The model under review builds one solid part; all positions refer to its coordinate system, in mm. A direction names the side the tool comes from. Give positions to 0.01 mm unless a question says otherwise; leave off trailing zeros. Loops run counter-clockwise (first coordinate to the right, second up) from the corner with the lowest first, then second, coordinate; pieces in that order, holes last. Notation, with made-up numbers: (-22, -33) - (4, -33) arc R17 ccw to (4, -25) - close; hole circle Ø1 at (22.5, -35). An arc over 180 degrees is marked (long way). Answer as a JSON object with one key per item and string values.
from build123d import *

# Parameters (mm, degrees)
SKETCH1_R           = 2.1
SKETCH1_R_2         = 2.6
BOSS_EXTRUDE1_DEPTH = 4


with BuildPart() as part:
    # Sketch1 → Boss-Extrude1 (new body)
    with BuildSketch(Plane(origin=(0, 0, 0), x_dir=(-1, 0, 0), z_dir=(0, 0, -1))):
        with BuildLine():
            Line((87.42535625, -29.106339063), (52.57464375, -20.393660937))
            ThreePointArc((52.57464375, -20.393660937), (47.11794562, -16.84635803), (45, -10.692235936))
            Line((45, -10.692235936), (45, -8))
            ThreePointArc((45, -8), (44.853553391, -7.646446609), (44.5, -7.5))
            Line((44.5, -7.5), (38, -7.5))
            ThreePointArc((38, -7.5), (37.646446609, -7.353553391), (37.5, -7))
            Line((37.5, -7), (37.5, 3))
            ThreePointArc((37.5, 3), (37.646446609, 3.353553391), (38, 3.5))
            Line((38, 3.5), (39.5, 3.5))
            ThreePointArc((39.5, 3.5), (39.853553391, 3.353553391), (40, 3))
            Line((40, 3), (40, -4.5))
            ThreePointArc((40, -4.5), (40.146446609, -4.853553391), (40.5, -5))
            Line((40.5, -5), (44.5, -5))
            ThreePointArc((44.5, -5), (44.853553391, -4.853553391), (45, -4.5))
            Line((45, -4.5), (45, 38.692235936))
            ThreePointArc((45, 38.692235936), (47.11794562, 44.84635803), (52.57464375, 48.393660937))
            Line((52.57464375, 48.393660937), (87.42535625, 57.106339063))
            ThreePointArc((87.42535625, 57.106339063), (92.88205438, 60.65364197), (95, 66.807764064))
            Line((95, 66.807764064), (95, 85))
            ThreePointArc((95, 85), (92.071067812, 92.071067812), (85, 95))
            Line((85, 95), (80.600023778, 95))
            ThreePointArc((80.600023778, 95), (75.38177505, 94.307249421), (70.525020806, 92.276988022))
            ThreePointArc((70.525020806, 92.276988022), (0, 73.215904175), (-70.525020806, 92.276988022))
            ThreePointArc((-70.525020806, 92.276988022), (-75.38177505, 94.307249421), (-80.600023778, 95))
            Line((-80.600023778, 95), (-85, 95))
            ThreePointArc((-85, 95), (-92.071067812, 92.071067812), (-95, 85))
            Line((-95, 85), (-95, 57.30993956))
            ThreePointArc((-95, 57.30993956), (-93.292887614, 51.721736358), (-88.754396995, 48.041471336))
            Line((-88.754396995, 48.041471336), (-51.245603005, 32.847708996))
            ThreePointArc((-51.245603005, 32.847708996), (-46.707112386, 29.167443975), (-45, 23.579240773))
            Line((-45, 23.579240773), (-45, -4.5))
            ThreePointArc((-45, -4.5), (-44.853553391, -4.853553391), (-44.5, -5))
            Line((-44.5, -5), (-40.5, -5))
            ThreePointArc((-40.5, -5), (-40.146446609, -4.853553391), (-40, -4.5))
            Line((-40, -4.5), (-40, 3))
            ThreePointArc((-40, 3), (-39.853553391, 3.353553391), (-39.5, 3.5))
            Line((-39.5, 3.5), (-38, 3.5))
            ThreePointArc((-38, 3.5), (-37.646446609, 3.353553391), (-37.5, 3))
            Line((-37.5, 3), (-37.5, -7))
            ThreePointArc((-37.5, -7), (-37.646446609, -7.353553391), (-38, -7.5))
            Line((-38, -7.5), (-44.5, -7.5))
            ThreePointArc((-44.5, -7.5), (-44.853553391, -7.646446609), (-45, -8))
            Line((-45, -8), (-45, -23.579240773))
            ThreePointArc((-45, -23.579240773), (-46.707112386, -29.167443975), (-51.245603005, -32.847708996))
            Line((-51.245603005, -32.847708996), (-88.754396995, -48.041471336))
            ThreePointArc((-88.754396995, -48.041471336), (-93.292887614, -51.721736358), (-95, -57.30993956))
            Line((-95, -57.30993956), (-95, -85))
            ThreePointArc((-95, -85), (-92.071067812, -92.071067812), (-85, -95))
            Line((-85, -95), (-80.600023778, -95))
            ThreePointArc((-80.600023778, -95), (-75.38177505, -94.307249421), (-70.525020806, -92.276988022))
            ThreePointArc((-70.525020806, -92.276988022), (0, -73.215904175), (70.525020806, -92.276988022))
            ThreePointArc((70.525020806, -92.276988022), (75.38177505, -94.307249421), (80.600023778, -95))
            Line((80.600023778, -95), (85, -95))
            ThreePointArc((85, -95), (92.071067812, -92.071067812), (95, -85))
            Line((95, -85), (95, -38.807764064))
            ThreePointArc((95, -38.807764064), (92.88205438, -32.65364197), (87.42535625, -29.106339063))
        make_face()
        with Locations((-85, -85)):
            Circle(SKETCH1_R, mode=Mode.SUBTRACT)
        with Locations((-85, 85)):
            Circle(SKETCH1_R, mode=Mode.SUBTRACT)
        with Locations((85, 85)):
            Circle(SKETCH1_R, mode=Mode.SUBTRACT)
        with Locations((85, -85)):
            Circle(SKETCH1_R, mode=Mode.SUBTRACT)
        with Locations((25, 19.006339063)):
            Circle(SKETCH1_R_2, mode=Mode.SUBTRACT)
        with Locations((25, -20.393660937)):
            Circle(SKETCH1_R_2, mode=Mode.SUBTRACT)
        with Locations((-25, -20.1)):
            Circle(SKETCH1_R_2, mode=Mode.SUBTRACT)
        with Locations((-25, 19.3)):
            Circle(SKETCH1_R_2, mode=Mode.SUBTRACT)
    extrude(amount=-BOSS_EXTRUDE1_DEPTH)


solid = part.part
Q1. Consider section C-C, the plane y = -77.5. State the section outline as (x, z) points.
Results:
{"outline": "(-95, 0) - (-34.37, 0) - (-34.37, 4) - (-95, 4) - close; (34.37, 0) - (95, 0) - (95, 4) - (34.37, 4) - close"}
Q2. Clearance check with flat-ended pins moving along their axes: pin 1 Ø1.2 at (y, z) = (4, 1) entering from +X; pin 2 Ø2 at (y, z) = (-10, 2) entering from -X; pin 3 Ø2 at (x, z) = (42, 2) entering from +Y. State where each tip first meets the part, or that it passes through.
Results:
{"pin 1": "stops at x = 45", "pin 2": "stops at x = -45", "pin 3": "stops at y = 79.98"}
Q3. The part is to be moulded in two halves that separate along Y. For faces 4 (the face through (1, 1, 4)), 5 (the face through (70.26, 40.55, 1.97)), 6 (the face through (-1.03, 73.22, 1.97)), say which applies: +Y half, -Y half, draft (parallel to the pull), parting line (faces both ways), or undercut.
Results:
{"face 4": "draft", "face 5": "undercut", "face 6": "+Y half"}
Q4. For faces 1 (the face through (22.6, 18.3, 2)), 2 (the face through (69.74, -40.34, 1.97)), 3 (the face through (-47.06, 44.77, 1.97)), list the 3-axis set-ups (+Z, -Z, +X, -X, +Y, -Y) from which the entire face can be reached by the end or side of a thin tool; tool diameter is ignored.
Results:
{"face 1": "+Z, -Z", "face 2": "+Z, -Z, +X", "face 3": "+Z, -Z, -X"}
Q5. To check wall thickness, follow probe 1 along Y at (x, z) = (85, 1.55); probe 2 along Y at (x, z) = (-25, 0.9); probe 3 along Y at (x, z) = (25, 2.1). State the ranges of each line that lie inside material, in increasing order. Write a range as [from, to].
Results:
{"probe 1": "y = [-95, -87.1], [-82.9, -46.52], [46.52, 82.9], [87.1, 95]", "probe 2": "y = [-75.47, -22.99], [-17.79, 16.41], [21.61, 75.47]", "probe 3": "y = [-75.47, -22.7], [-17.5, 16.7], [21.9, 75.47]"}
Q6. Consider section A-A, the plane x = -63.5. State the section outline as (y, z) points (3 decimals).
Results:
{"outline": "(-88.445, 0) - (-23.125, 0) - (-23.125, 4) - (-88.445, 4) - close; (51.125, 0) - (88.445, 0) - (88.445, 4) - (51.125, 4) - close"}
Q7. Consider section B-B, the plane x = -25. State the section outline as (y, z) points.
Results:
{"outline": "(-75.47, 0) - (-22.99, 0) - (-22.99, 4) - (-75.47, 4) - close; (-17.79, 0) - (16.41, 0) - (16.41, 4) - (-17.79, 4) - close; (21.61, 0) - (75.47, 0) - (75.47, 4) - (21.61, 4) - close"}
Q8. Consider section D-D, the plane z = 2.65. State how many separate pieces and enclosed holes the cut face has, plus the area to 3 significant figures.
Results:
{"separate pieces": "1", "enclosed holes": "8", "area": "23,400 mm^2"}
